```python
from build123d import *

# Parameters (mm, degrees)
SKETCH2_R             = 2.35
BOSS_EXTRUDE1_DEPTH   = 2.5
BOSS_EXTRUDE1_2_DEPTH = 2.5
SKETCH2_W             = 4.6228
SKETCH2_H             = 4.6228
BOSS_EXTRUDE1_3_DEPTH = 2.5
BOSS_EXTRUDE1_4_DEPTH = 2.5
BOSS_EXTRUDE2_DEPTH   = 6.075
SKETCH6_R             = 2.35
CUT_EXTRUDE1_DEPTH    = 201.98763799
SKETCH4_R             = 7.5
SKETCH4_R_2           = 2.35
BOSS_EXTRUDE4_DEPTH   = 6
FILLET2_R             = 2.5
FILLET3_R             = 8
SKETCH7_R             = 2.35
CUT_EXTRUDE2_DEPTH    = 215.594236042
FILLET4_R             = 1.5
FILLET5_R             = 0.75


with BuildPart() as part:
    # Sketch2 → Boss-Extrude1 (new body)
    with BuildSketch(Plane.XY):
        with Locations((44.45, 184.15)):
            Circle(SKETCH2_R)
    extrude(amount=BOSS_EXTRUDE1_DEPTH)


with BuildPart() as body_2:
    # Sketch2 → Boss-Extrude1 2 (new body)
    with BuildSketch(Plane.XY):
        with Locations((57.15, 171.45)):
            Circle(SKETCH2_R)
    extrude(amount=BOSS_EXTRUDE1_2_DEPTH)


with BuildPart() as body_3:
    # Sketch2 → Boss-Extrude1 3 (new body)
    with BuildSketch(Plane.XY):
        with Locations((57.15, 184.15)):
            Rectangle(SKETCH2_W, SKETCH2_H)
    extrude(amount=BOSS_EXTRUDE1_3_DEPTH)



with BuildPart() as body_4:
    # Sketch2 → Boss-Extrude1 4 (new body)
    with BuildSketch(Plane.XY):
        with Locations((44.45, 171.45)):
            Rectangle(SKETCH2_W, SKETCH2_H)
    extrude(amount=BOSS_EXTRUDE1_4_DEPTH)


with BuildPart() as body_3_1:
    add(body_3.part)

    add(body_4.part)  # Boss-Extrude2 merges body 4
    # Sketch3 → Boss-Extrude2 (add)
    with BuildSketch(Plane.XY):
        with BuildLine():
            Line((63.5, 186.4614), (63.5, 165.1))
            Line((63.5, 165.1), (38.1, 165.1))
            Line((38.1, 165.1), (38.1, 190.5))
            Line((38.1, 190.5), (59.4614, 190.5))
            ThreePointArc((59.4614, 190.5), (61.102474131, 188.102474131), (63.5, 186.4614))
        make_face()
    extrude(amount=-BOSS_EXTRUDE2_DEPTH)


with BuildPart() as cut_extrude1_tool:
    # Sketch6 → Cut-Extrude1 (new, through all)
    with BuildSketch(Plane.XY.offset(2.5)):
        with Locations((44.45, 184.15)):
            Circle(SKETCH6_R)
        with Locations((57.15, 171.45)):
            Circle(SKETCH6_R)
    extrude(amount=-CUT_EXTRUDE1_DEPTH)


with BuildPart() as part_1:
    add(part.part)

    # Cut-Extrude1: cut by cut_extrude1_tool
    add(cut_extrude1_tool.part, mode=Mode.SUBTRACT)


with BuildPart() as body_2_1:
    add(body_2.part)

    # Cut-Extrude1: cut by cut_extrude1_tool
    add(cut_extrude1_tool.part, mode=Mode.SUBTRACT)


with BuildPart() as body_3_2:
    add(body_3_1.part)

    # Cut-Extrude1: cut by cut_extrude1_tool
    add(cut_extrude1_tool.part, mode=Mode.SUBTRACT)

    # Sketch4 → Boss-Extrude4 (add)
    # profile 1 of 3: a face of its own
    with BuildSketch(Plane(origin=(0, 0, -6.075), x_dir=(-1, 0, 0), z_dir=(0, 0, -1))):
        with Locations((-66.681980515, 193.681980515)):
            Circle(SKETCH4_R)
        with Locations((-66.681980515, 193.681980515)):
            Circle(SKETCH4_R_2, mode=Mode.SUBTRACT)
    # profile 2 of 3: a face of its own
    with BuildSketch(Plane(origin=(0, 0, -6.075), x_dir=(-1, 0, 0), z_dir=(0, 0, -1))):
        with BuildLine():
            Line((-38.1, 190.5), (-59.4614, 190.5))
            ThreePointArc((-59.4614, 190.5), (-61.102474131, 188.102474131), (-63.5, 186.4614))
            Line((-63.5, 186.4614), (-63.5, 165.1))
            Line((-63.5, 165.1), (-38.1, 165.1))
            Line((-38.1, 165.1), (-38.1, 190.5))
        make_face()
    # profile 3 of 3: a face of its own
    with BuildSketch(Plane(origin=(0, 0, -6.075), x_dir=(-1, 0, 0), z_dir=(0, 0, -1))):
        with BuildLine():
            ThreePointArc((-63.5, 186.4614), (-61.102474131, 188.102474131), (-59.4614, 190.5))
            Line((-59.4614, 190.5), (-59.890441662, 190.5))
            ThreePointArc((-59.890441662, 190.5), (-61.378679656, 188.378679656), (-63.5, 186.890441662))
            Line((-63.5, 186.890441662), (-63.5, 186.4614))
        make_face()
    extrude(amount=BOSS_EXTRUDE4_DEPTH)

    # Fillet2
    fillet2_edges = [body_3_2.edges().sort_by_distance(p)[0] for p in [
        (63.5, 186.890441662, -9.075),
    ]]
    fillet(fillet2_edges, radius=FILLET2_R)

    # Fillet3
    # the kernel refuses this fillet: 8 mm, written as the material it adds along each edge
    with BuildSketch(Plane(origin=(59.890441662, 190.5, 13.776565592), x_dir=(-1, 0, 0), z_dir=(0, 0, -1))) as fillet3_piece_1_section:
        with BuildLine():
            CenterArc((7.940626237, 8), FILLET3_R, 198.10985807, 71.89014193)
            ThreePointArc((0.336928126, 5.513280266), (0.694495171, 2.724493268), (0, 0))
            Line((0, 0), (7.940626237, 0))
        make_face()
    fillet3_piece_1 = extrude(amount=25.851565592, mode=Mode.PRIVATE)
    fillet3_piece_1 = fillet3_piece_1 - Plane(origin=(66.681980515, 193.681980515, -3.0375), x_dir=(-0.9150847933660875, -0.40326147962599274, 0), z_dir=(0, 0, 1)) * Cylinder(7.8906136, 84, mode=Mode.PRIVATE)
    fillet3_piece_1 = split(fillet3_piece_1, bisect_by=Plane(origin=(57.125105601, 191.419685935, 0), z_dir=(0, 0, -1)), keep=Keep.TOP, mode=Mode.PRIVATE)
    fillet3_piece_1 = split(fillet3_piece_1, bisect_by=Plane(origin=(57.125105601, 191.419685935, -6.075), z_dir=(0, 0, 1)), keep=Keep.TOP, mode=Mode.PRIVATE)
    add(fillet3_piece_1)
    with BuildSketch(Plane(origin=(59.890441662, 190.5, -6.075), x_dir=(-1, 0, 0), z_dir=(0, 0, -1))) as fillet3_piece_2_section:
        with BuildLine():
            CenterArc((7.940626237, 8), FILLET3_R, 198.10985807, 71.89014193)
            ThreePointArc((0.336928126, 5.513280266), (0.694495171, 2.724493268), (0, 0))
            Line((0, 0), (7.940626237, 0))
        make_face()
    fillet3_piece_2 = extrude(amount=6, mode=Mode.PRIVATE)
    fillet3_piece_2 = fillet3_piece_2 - Plane(origin=(66.681980515, 193.681980515, -9.075), x_dir=(-0.9150847933660875, -0.40326147962599274, 0), z_dir=(0, 0, 1)) * Cylinder(7.8906136, 44, mode=Mode.PRIVATE)
    add(fillet3_piece_2)
    with BuildSketch(Plane(origin=(59.890441662, 190.5, -6.075), x_dir=(-1, 0, 0), z_dir=(0, 0, -1))) as fillet3_piece_3_section:
        with BuildLine():
            CenterArc((7.940626237, 8), FILLET3_R, 198.10985807, 71.89014193)
            ThreePointArc((0.336928126, 5.513280266), (0.694495171, 2.724493268), (0, 0))
            Line((0, 0), (7.940626237, 0))
        make_face()
    fillet3_piece_3 = extrude(amount=6, mode=Mode.PRIVATE)
    fillet3_piece_3 = fillet3_piece_3 & Plane(origin=(66.681980515, 193.681980515, -9.075), x_dir=(-0.9150847933660875, -0.40326147962599274, 0), z_dir=(0, 0, 1)) * Cylinder(7.8906136, 44, mode=Mode.PRIVATE)
    add(fillet3_piece_3)

    # Sketch7 → Cut-Extrude2 (cut, through all)
    with BuildSketch(Plane.XY.offset(-6.075)):
        with Locations((44.45, 184.15)):
            Circle(SKETCH7_R)
        with Locations((57.15, 171.45)):
            Circle(SKETCH7_R)
    extrude(amount=-CUT_EXTRUDE2_DEPTH, mode=Mode.SUBTRACT)

    # Fillet4
    fillet4_edges = [body_3_2.edges().sort_by_distance(p)[0] for p in [
        (58.824977937, 194.409506089, -3.0375),
    ]]
    fillet(fillet4_edges, radius=FILLET4_R)

    # Fillet5
    fillet5_edges = [body_3_2.edges().sort_by_distance(p)[0] for p in [
        (46.7614, 173.7614, 1.25),
        (42.1386, 173.7614, 1.25),
        (42.1386, 169.1386, 1.25),
        (46.7614, 169.1386, 1.25),
        (59.4614, 181.8386, 1.25),
        (54.8386, 181.8386, 1.25),
        (54.8386, 186.4614, 1.25),
        (59.4614, 186.4614, 1.25),
    ]]
    fillet(fillet5_edges, radius=FILLET5_R)


solid = body_3_2.part
```
Geometry check sheet. Reference: the model listing, model coordinates, mm. A direction names the side the tool comes from. Round coordinates to 2 decimals unless told otherwise and drop trailing zeros. Loops run counter-clockwise (first coordinate to the right, second up) from the corner with the lowest first, then second, coordinate; pieces in that order, holes last. Notation, with made-up numbers: (-3, 84.25) - (15, 84.25) arc R12 ccw to (15, 102.25) - close; hole circle Ø9 at (-37, 7). An arc over 180 degrees is marked (long way). Write each question's results on one line, items separated by ' | '. Start each with the question number.
Q1. Gauge pin test, flat ends, axial feed: P1, Ø2, axis at y = 172, z = 1.5, coming from the -X side; P2, Ø2, axis at x = 48.5, z = -7, coming from the +Y side; P3, Ø7.5, axis at x = 66.68, y = 193.68, coming from the +Z side (3 decimals). Record the tip position at first contact, or that the pin passes through.
Q2. Cross-section at A-A on y = 171.45. Enter the section's corners in (x, z) (3 decimals), and give its area (3 significant figures).
Q3. Release check for a two-part mould opening along X. For faces 5 (the cylindrical face through (43.941, 181.856, -5.953)), 6 (the cylindrical face through (55.762, 191.467, -7.295)), 7 (the flat face through (57, 184, 2.5)), 8 (the flat face through (46.761, 171, 1)) record: +X half, -X half, draft (parallel to the pull), parting line (faces both ways), or undercut.
Q4. Cross-section at B-B on x = 44.45. Enter the section's corners in (y, z) (3 decimals).
Q5. Access from +Z, -Z, +X, -X, +Y, -Y to the whole of each face (thin tool, end or side, straight path). Record for faces 1 (the flat face through (57, 186.461, 1)), 2 (the flat face through (69.2, 193.7, -6.075)), 3 (the flat face through (44, 169.139, 1)), 4 (the flat face through (45, 190.5, -6)).
Q6. Thickness scan on line 1 (X direction, y = 171.45, z = -4); line 2 (Y direction, x = 44.45, z = -4.75); line 3 (Z direction, x = 62, y = 199.5) (3 decimals). Record the ranges inside material, lowest first. Write a range as [from, to].
Q7. Cross-section at C-C on z = -7. Enter the section's corners in (x, y), and give its area (3 significant figures).
Q8. Cross-section at D-D on y = 178. Enter the section's corners in (x, z) (3 decimals).
Answers below:
1) P1: stops at x = 42.14 | P2: stops at y = 190.5 | P3: stops at z = -6.075
2) outline: (38.1, -12.075) - (54.8, -12.075) - (54.8, 0) - (46.761, 0) - (46.761, 2.5) - (42.139, 2.5) - (42.139, 0) - (38.1, 0) - close; (59.5, -12.075) - (63.5, -12.075) - (63.5, 0) - (59.5, 0) - close | area: 262 mm²
3) face 5: undercut | face 6: -X half | face 7: draft | face 8: +X half
4) outline: (165.1, -12.075) - (181.8, -12.075) - (181.8, 0) - (173.761, 0) - (173.761, 2.5) - (169.139, 2.5) - (169.139, 0) - (165.1, 0) - close; (186.5, -12.075) - (190.5, -12.075) - (190.5, 0) - (186.5, 0) - close
5) face 1: +Z, +X, -X, +Y | face 2: +Z, +X, +Y | face 3: +Z, +X, -X, -Y | face 4: +Z, -Z, -X, +Y
6) line 1: x = [38.1, 54.8], [59.5, 63.5] | line 2: y = [165.1, 181.8], [186.5, 190.5] | line 3: z = [-12.075, -6.075]
7) outline: (38.1, 165.1) - (63.5, 165.1) - (63.5, 183.71) arc R2.5 cw to (66.17, 186.2) arc R7.5 ccw (long way) to (59.55, 196.01) arc R8 cw to (51.95, 190.5) - (38.1, 190.5) - close; hole circle Ø4.7 at (44.45, 184.15); hole circle Ø4.7 at (57.15, 171.45); hole circle Ø4.7 at (66.68, 193.68) | area: 774 mm²
8) outline: (38.1, -12.075) - (63.5, -12.075) - (63.5, 0) - (38.1, 0) - close
